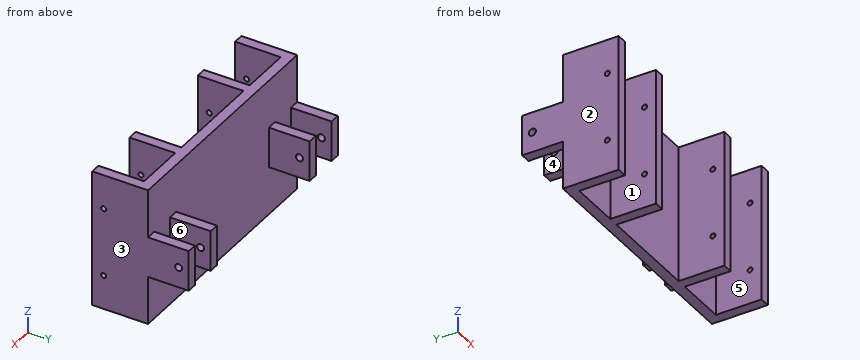
```python
from build123d import *

# Parameters (mm, degrees)
BOSS_EXTRUDE1_DEPTH     = 135
SKETCH3_W               = 10
SKETCH3_H               = 135
BOSS_EXTRUDE2_DEPTH     = 45
CUT_EXTRUDE1_DEPTH      = 230
CUT_EXTRUDE1_DEPTH_BACK = 10
SKETCH4_W               = 10
SKETCH4_H               = 20
BOSS_EXTRUDE3_DEPTH     = 40
CUT_EXTRUDE2_DEPTH      = 281.802421642
CUT_EXTRUDE2_DEPTH_BACK = 240


with BuildPart() as part:
    # Sketch1 → Boss-Extrude1 (new body)
    with BuildSketch(Plane.XY):
        Polygon((-120, 0), (120, 0), (120, -55), (110, -55), (110, -10), (-110, -10), (-110, -55), (-120, -55), align=None)
    extrude(amount=BOSS_EXTRUDE1_DEPTH)

    # Sketch3 → Boss-Extrude2 (add)
    with BuildSketch(Plane.XZ.offset(10)):
        with Locations((55, 67.5)):
            Rectangle(SKETCH3_W, SKETCH3_H)
        with Locations((-55, 67.5)):
            Rectangle(SKETCH3_W, SKETCH3_H)
    extrude(amount=BOSS_EXTRUDE2_DEPTH)

    # Sketch2 → Cut-Extrude1 (cut, two sides: drawn at the far end of the back side and taken through both)
    with BuildSketch(Plane.ZY.offset(-110).offset(-CUT_EXTRUDE1_DEPTH_BACK)):
        with BuildLine():
            ThreePointArc((31.25, -43.75), (33.75, -46.25), (36.25, -43.75))
            Line((36.25, -43.75), (33.75, -43.75))
            Line((33.75, -43.75), (31.25, -43.75))
        make_face()
        with BuildLine():
            Line((33.75, -43.75), (36.25, -43.75))
            ThreePointArc((36.25, -43.75), (33.75, -41.25), (31.25, -43.75))
            Line((31.25, -43.75), (33.75, -43.75))
        make_face()
        with BuildLine():
            Line((98.75, -43.75), (101.25, -43.75))
            Line((101.25, -43.75), (103.75, -43.75))
            ThreePointArc((103.75, -43.75), (101.25, -41.25), (98.75, -43.75))
        make_face()
        with BuildLine():
            Line((103.75, -43.75), (101.25, -43.75))
            Line((101.25, -43.75), (98.75, -43.75))
            ThreePointArc((98.75, -43.75), (101.25, -46.25), (103.75, -43.75))
        make_face()
    extrude(amount=CUT_EXTRUDE1_DEPTH + CUT_EXTRUDE1_DEPTH_BACK, mode=Mode.SUBTRACT)

    # Sketch4 → Boss-Extrude3 (add)
    with BuildSketch(Plane(origin=(0, 0, 0), x_dir=(1, 0, 0), z_dir=(0, 1, 0))):
        with Locations((-115, -57.5)):
            Rectangle(SKETCH4_W, SKETCH4_H)
        with Locations((-115, -77.5)):
            Rectangle(SKETCH4_W, SKETCH4_H)
        with Locations((-79.6, -77.5)):
            Rectangle(SKETCH4_W, SKETCH4_H)
        with Locations((-79.6, -57.5)):
            Rectangle(SKETCH4_W, SKETCH4_H)
        with Locations((79.6, -57.5)):
            Rectangle(SKETCH4_W, SKETCH4_H)
        with Locations((79.6, -77.5)):
            Rectangle(SKETCH4_W, SKETCH4_H)
        with Locations((115, -77.5)):
            Rectangle(SKETCH4_W, SKETCH4_H)
        with Locations((115, -57.5)):
            Rectangle(SKETCH4_W, SKETCH4_H)
    extrude(amount=BOSS_EXTRUDE3_DEPTH)

    # Sketch5 → Cut-Extrude2 (cut, two sides: drawn at the far end of the back side and taken through both)
    with BuildSketch(Plane(origin=(120, 0, 0), x_dir=(0, 0, -1), z_dir=(1, 0, 0)).offset(-CUT_EXTRUDE2_DEPTH_BACK)):
        with BuildLine():
            ThreePointArc((-67.5, 33.5), (-71, 30), (-67.5, 26.5))
            Line((-67.5, 26.5), (-67.5, 30))
            Line((-67.5, 30), (-67.5, 33.5))
        make_face()
        with BuildLine():
            Line((-67.5, 30), (-67.5, 26.5))
            ThreePointArc((-67.5, 26.5), (-65.025126266, 27.525126266), (-64, 30))
            ThreePointArc((-64, 30), (-65.025126266, 32.474873734), (-67.5, 33.5))
            Line((-67.5, 33.5), (-67.5, 30))
        make_face()
    extrude(amount=CUT_EXTRUDE2_DEPTH + CUT_EXTRUDE2_DEPTH_BACK, mode=Mode.SUBTRACT)


solid = part.part
```
Build history of the part. All positions in model axes, mm. Face numbers are marked on the shaded views. A direction names the side the tool comes from. Round coordinates to 2 decimals unless told otherwise and drop trailing zeros. Write each loop counter-clockwise with the first axis right and the second up, starting at its lowest first coordinate (ties: lowest second). Pieces come first, ordered by that corner, then holes.
1) Band-saw the part on D-D, the plane z = 121. List the corners of the cut face in (x, y).
2) 3-axis set-ups, long thin cutter, end or side, ignore diameter. For the marked faces 5 and 6: which of +Z, -Z, +X, -X, +Y, -Y reach the whole face in a straight line?
3) Band-saw the part on B-B, the plane z = 33.75. Give the number of separate pieces and of enclosed holes in the cut face, and give its area (3 significant figures).
4) Drill centre lines: probe 1 along X at (y, z) = (-24.5, 122.5); probe 2 along X at (y, z) = (13.5, 55.5); probe 3 along Z at (x, y) = (-117.75, -43.75). Where is each one in solid material? Low to high.
5) Band-saw the part on A-A, the plane y = -36.5. List the corners of the cut face in (x, z), and give its area (3 significant figures).
6) Mould opens along X. For the marked faces 1, 2, 3 and 4 say: +X half, -X half, draft (parallel to the pull), parting line (faces both ways), or undercut.
7) Pin check, flat tips, straight feed: pin 1 (3 mm diameter, centred on x = 45.5, z = 95.5, fed in from +Y); pin 2 (3 mm diameter, centred on x = -80.5, y = 23.5, fed in from -Z); pin 3 (3 mm diameter, centred on x = 81, y = 12, fed in from +Z). Stop position of each tip, or through.
8) Band-saw the part on C-C, the plane x = -53. List the corners of the cut face in (y, z), and give its area (3 significant figures).
Ans:
1. outline: (-120, -55) - (-110, -55) - (-110, -10) - (-60, -10) - (-60, -55) - (-50, -55) - (-50, -10) - (50, -10) - (50, -55) - (60, -55) - (60, -10) - (110, -10) - (110, -55) - (120, -55) - (120, 0) - (-120, 0) - close
2. face 5: +Z, -Z, -Y
2. face 6: +Z, -Z, +Y
3. separate pieces: 5
3. enclosed holes: 0
3. area: 4,000 mm2
4. probe 1: x = -120 to -110, -60 to -50, 50 to 60, 110 to 120
4. probe 2: x = -120 to -110, -84.6 to -74.6, 74.6 to 84.6, 110 to 120
4. probe 3: z = 0 to 31.25, 36.25 to 98.75, 103.75 to 135
5. outline: (-120, 0) - (-110, 0) - (-110, 135) - (-120, 135) - close; (-60, 0) - (-50, 0) - (-50, 135) - (-60, 135) - close; (50, 0) - (60, 0) - (60, 135) - (50, 135) - close; (110, 0) - (120, 0) - (120, 135) - (110, 135) - close
5. area: 5,400 mm2
6. face 1: undercut
6. face 2: -X half
6. face 3: +X half
6. face 4: undercut
7. pin 1: stops at y = 0
7. pin 2: stops at z = 47.5
7. pin 3: stops at z = 87.5
8. outline: (-55, 0) - (0, 0) - (0, 135) - (-55, 135) - close; hole circle Ø5 at (-43.75, 33.75); hole circle Ø5 at (-43.75, 101.25)
8. area: 7,390 mm2
